Here's how the part is built. I have some questions about the finished solid (model axes, mm). A direction names the side the tool comes from. Round coordinates to 2 decimals unless told otherwise and drop trailing zeros. Order: outer loops, then holes, each group sorted by start corner. A loop starts at its lowest first (then second) coordinate and runs counter-clockwise, first axis right, second up.
```python
from build123d import *

# Parameters (mm, degrees)
F0_R     = 9.525
F0_R_2   = 12.7
F1_DEPTH = 12.7
F0_R_3   = 6.35
F2_DEPTH = 38.1


with BuildPart() as f1:
    # F0 (on Front) → F1 (new body)
    with BuildSketch(Plane.XZ):
        with BuildLine():
            ThreePointArc((19.0800315969, 33.5443825636), (17.7775003101, 30.0599167658), (14.3667655142, 28.575))
            Line((14.3667655142, 28.575), (-14.3667655142, 28.575))
            ThreePointArc((-14.3667655142, 28.575), (-18.3550358696, 30.4875726696), (-19.0500754755, 34.8557707639))
            ThreePointArc((-19.0500754755, 34.8557707639), (-50.7653853614, 66.6749811311), (-82.55, 34.925))
            Line((-82.55, 34.925), (-82.55, 7.4563898))
            ThreePointArc((-82.55, 7.4563898), (-83.6234833627, 4.4443203287), (-86.36, 2.79011184))
            ThreePointArc((-86.36, 2.79011184), (-101.6, -15.875), (-86.36, -34.54011184))
            Line((-86.36, -34.54011184), (-53.975, -34.54011184))
            ThreePointArc((-53.975, -34.54011184), (-47.2398079092, -37.3299197492), (-44.45, -44.06511184))
            Line((-44.45, -44.06511184), (-44.45, -50.8))
            ThreePointArc((-44.45, -50.8), (-41.6601920908, -57.5351920908), (-34.925, -60.325))
            Line((-34.925, -60.325), (-19.05, -60.325))
            Line((-19.05, -60.325), (-19.05, -47.625))
            ThreePointArc((-19.05, -47.625), (-13.4703841816, -34.1546158184), (0, -28.575))
            ThreePointArc((0, -28.575), (13.4703841816, -34.1546158184), (19.05, -47.625))
            Line((19.05, -47.625), (19.05, -60.325))
            Line((19.05, -60.325), (34.925, -60.325))
            ThreePointArc((34.925, -60.325), (41.6601920908, -57.5351920908), (44.45, -50.8))
            Line((44.45, -50.8), (44.45, -44.06511184))
            ThreePointArc((44.45, -44.06511184), (47.2398079092, -37.3299197492), (53.975, -34.54011184))
            Line((53.975, -34.54011184), (86.36, -34.54011184))
            ThreePointArc((86.36, -34.54011184), (101.6, -15.875), (86.36, 2.79011184))
            ThreePointArc((86.36, 2.79011184), (83.6234833627, 4.4443203287), (82.55, 7.4563898))
            Line((82.55, 7.4563898), (82.55, 34.925))
            ThreePointArc((82.55, 34.925), (50.1095279871, 66.6674912129), (19.0800315969, 33.5443825636))
        make_face()
        with Locations((-82.55, -15.875)):
            Circle(F0_R, mode=Mode.SUBTRACT)
        Circle(F0_R_2, mode=Mode.SUBTRACT)
        with Locations((82.55, -15.875)):
            Circle(F0_R, mode=Mode.SUBTRACT)
        with Locations((-50.8, 34.925)):
            Circle(F0_R_2, mode=Mode.SUBTRACT)
        with Locations((50.8, 34.925)):
            Circle(F0_R_2, mode=Mode.SUBTRACT)
    extrude(amount=F1_DEPTH)

    # F0 (on Front) → F2 (join)
    with BuildSketch(Plane.XZ):
        with Locations((-82.55, -15.875)):
            Circle(F0_R)
        with Locations((-82.55, -15.875)):
            Circle(F0_R_3, mode=Mode.SUBTRACT)
        with Locations((82.55, -15.875)):
            Circle(F0_R)
        with Locations((82.55, -15.875)):
            Circle(F0_R_3, mode=Mode.SUBTRACT)
    extrude(amount=F2_DEPTH)


solid = f1.part
```
1. I need wall thicknesses on probe 1 along X at (y, z) = (-11.5, 34); probe 2 along X at (y, z) = (-15, -10); probe 3 along Z at (x, y) = (82.55, -19) (3 decimals). Which ranges of each line are inside material? Lowest first, please.
Evaluation:
probe 1: x = -82.55 to -63.47, -38.13 to -19.25, 19.06 to 38.13, 63.47 to 82.55
probe 2: x = -90.05 to -84.96, -80.14 to -75.05, 75.05 to 80.14, 84.96 to 90.05
probe 3: z = -25.4 to -22.225, -9.525 to -6.35
2. If we section it at B-B, the plane z = 55.5: Write out the boundary of the cut face in (x, y), and give its area (3 significant figures).
Evaluation:
outline: (-74.98, -12.7) - (-26.62, -12.7) - (-26.62, 0) - (-74.98, 0) - close; (26.62, -12.7) - (74.98, -12.7) - (74.98, 0) - (26.62, 0) - close
area: 1,230 mm2
3. If we mould it in two halves opening along Z, with no side actions, what happens to faces 5 (the cylindrical face through (-38.686, -6.261, 38.74)), 6 (the flat face through (-80.6, -38.1, -22.1)), 7 (the flat face through (-70, -6, -34.54))? For each: released by +Z, released by -Z, zero draft, split by the parting line, or undercut.
Evaluation:
face 5: undercut
face 6: zero draft
face 7: released by -Z
4. If we section it at D-D, the plane y = -10.5: State how many separate pieces and enclosed holes the cut face has, and give its area (3 significant figures).
Evaluation:
separate pieces: 1
enclosed holes: 5
area: 15,000 mm2
5. I'm going to push flat-ended pins straight in: P1, Ø2, axis at x = 4.5, z = 22, coming from the -Y side; P2, Ø10, axis at y = -5, z = 53.5, coming from the -X side; P3, Ø14, axis at y = -8, z = -57, coming from the -X side; P4, Ø20.5, axis at x = 50.8, z = 34.925, coming from the -Y side. Where does each tip first touch, or does it pass through?
Evaluation:
P1: stops at y = -12.7
P2: stops at x = -79.5
P3: stops at x = -44.45
P4: passes through
6. If we section it at C-C, the plane z = 41: Write out the boundary of the cut face in (x, y).
Evaluation:
outline: (-81.96, -12.7) - (-61.95, -12.7) - (-61.95, 0) - (-81.96, 0) - close; (-39.65, -12.7) - (-19.64, -12.7) - (-19.64, 0) - (-39.65, 0) - close; (19.64, -12.7) - (39.65, -12.7) - (39.65, 0) - (19.64, 0) - close; (61.95, -12.7) - (81.96, -12.7) - (81.96, 0) - (61.95, 0) - close
7. On a 3-axis mill with a long thin cutter (end or side, diameter ignored), from which of +Z, -Z, +X, -X, +Y, -Y can I reach the whole of each face in a straight line? I mean faces 1 (the flat face through (-82.55, -6, 21)), 2 (the flat face through (0, -6, 28.575)), 3 (the flat face through (-27, -6, -60.325)), 4 (the cylindrical face through (-18.32, -6.26, 30.44)). Say none if no direction works.
Evaluation:
face 1: +Z, -X, +Y, -Y
face 2: +Z, +Y, -Y
face 3: -Z, +X, -X, +Y, -Y
face 4: +Y, -Y
8. If we section it at A-A, the plane x = 8: Write out the boundary of the cut face in (y, z) (3 decimals).
Evaluation:
outline: (-12.7, -30.336) - (0, -30.336) - (0, -9.864) - (-12.7, -9.864) - close; (-12.7, 9.864) - (0, 9.864) - (0, 28.575) - (-12.7, 28.575) - close
